Design review of the part built by this model. Coordinates are the model's own, in mm. A direction names the side the tool comes from. Give positions to 0.01 mm unless a question says otherwise; leave off trailing zeros. Order: outer loops, then holes, each group sorted by start corner. A loop starts at its lowest first (then second) coordinate and runs counter-clockwise, first axis right, second up. Notation, with made-up numbers: (61.25, 74) -> (105.25, 74) arc R19 ccw to (105.25, 107) -> close; hole circle Ø9 at (24, -11.5). An arc over 180 degrees is marked (long way). Return JSON: item names as keys, results as strings.
```python
from build123d import *
from build123d.topology import SkipClean

# Parameters (mm, degrees)
SKETCH2_R           = 31.369
BOSS_EXTRUDE1_DEPTH = 25.4
BOSS_EXTRUDE2_START = 125.476
BOSS_EXTRUDE2_DEPTH = 125.476
BOSS_EXTRUDE3_DEPTH = 49.022
SKETCH8_W           = 125.476
SKETCH8_H           = 49.022
BOSS_EXTRUDE4_DEPTH = 35.052
SKETCH9_W           = 125.476
SKETCH9_H           = 49.022
BOSS_EXTRUDE5_DEPTH = 35.052
SKETCH10_W          = 125.476
SKETCH10_H          = 35.052
BOSS_EXTRUDE6_DEPTH = 38.1
SKETCH12_W          = 125.476
SKETCH12_H          = 60.452
BOSS_EXTRUDE7_DEPTH = 52.324


with BuildPart() as part:
    # Sketch2 → Boss-Extrude1 (new body)
    with BuildSketch(Plane.YZ):
        with Locations(Location((0, 0, 0), (0, 0, 270))):
            Circle(SKETCH2_R)
    extrude(amount=BOSS_EXTRUDE1_DEPTH)

    # Sketch4 → Boss-Extrude2 (add)
    with SkipClean():  # the faces are left unmerged after this step: merging them gives an invalid solid
        with BuildSketch(Plane(origin=(0, 0, 0), x_dir=(0, -1, 0), z_dir=(-1, 0, 0)).offset(BOSS_EXTRUDE2_START)):
            with BuildLine():
                Line((31.369, 0), (31.369, 76.2))
                Line((31.369, 76.2), (-31.369, 76.2))
                Line((-31.369, 76.2), (-31.369, 0))
                ThreePointArc((-31.369, 0), (0, -31.369), (31.369, 0))
            make_face()
        extrude(amount=-BOSS_EXTRUDE2_DEPTH)

    # Sketch5 → Boss-Extrude3 (add)
    with SkipClean():  # the faces are left unmerged after this step: merging them gives an invalid solid
        with BuildSketch(Plane.XY.offset(76.2)):
            Polygon((0, 0), (0, 62.747251031), (-125.476, 62.747251031), (-125.476, -62.747251031), (0, -62.747251031), align=None)
        extrude(amount=BOSS_EXTRUDE3_DEPTH)

    # Sketch8 → Boss-Extrude4 (add)
    with SkipClean():  # the faces are left unmerged after this step: merging them gives an invalid solid
        with BuildSketch(Plane(origin=(0, 62.747251031, 0), x_dir=(-1, 0, 0), z_dir=(0, 1, 0))):
            with Locations((62.738, 100.711)):
                Rectangle(SKETCH8_W, SKETCH8_H)
        extrude(amount=BOSS_EXTRUDE4_DEPTH)

    # Sketch9 → Boss-Extrude5 (add)
    with SkipClean():  # the faces are left unmerged after this step: merging them gives an invalid solid
        with BuildSketch(Plane.XZ.offset(62.747251031)):
            with Locations((-62.738, 100.711)):
                Rectangle(SKETCH9_W, SKETCH9_H)
        extrude(amount=BOSS_EXTRUDE5_DEPTH)

    # Sketch10 → Boss-Extrude6 (add)
    with SkipClean():  # the faces are left unmerged after this step: merging them gives an invalid solid
        with BuildSketch(Plane.XY.offset(125.222)):
            with Locations((-62.738, 80.273251031)):
                Rectangle(SKETCH10_W, SKETCH10_H)
            with Locations((-62.738, -80.273251031)):
                Rectangle(SKETCH10_W, SKETCH10_H)
        extrude(amount=BOSS_EXTRUDE6_DEPTH)

    # Sketch12 → Boss-Extrude7 (add)
    with SkipClean():  # the faces are left unmerged after this step: merging them gives an invalid solid
        with BuildSketch(Plane.XY.offset(163.322)):
            with Locations((-62.738, 67.573251031)):
                Rectangle(SKETCH12_W, SKETCH12_H)
            with Locations((-62.738, -67.573251031)):
                Rectangle(SKETCH12_W, SKETCH12_H)
        extrude(amount=BOSS_EXTRUDE7_DEPTH)


solid = part.part
```
Item 1: Wall thickness on L1, parallel to Y at x = -32.5, z = 131.5; L2, parallel to Z at x = -24.5, y = 48.5; L3, parallel to Z at x = -113.5, y = -68.5: over which ranges is each line inside the solid? List them lowest first. Write a range as [from, to].
Result set:
{"L1": "y = [-97.8, -62.75], [62.75, 97.8]", "L2": "z = [76.2, 125.22], [163.32, 215.65]", "L3": "z = [76.2, 215.65]"}
Item 2: Add section C-C (x = -92). Give the boundary of the cut face in (y, z), plus the area to 3 significant figures.
Result set:
{"outline": "(-97.8, 76.2) -> (-31.37, 76.2) -> (-31.37, 0) arc R31.37 ccw to (31.37, 0) -> (31.37, 76.2) -> (97.8, 76.2) -> (97.8, 215.65) -> (37.35, 215.65) -> (37.35, 163.32) -> (62.75, 163.32) -> (62.75, 125.22) -> (-62.75, 125.22) -> (-62.75, 163.32) -> (-37.35, 163.32) -> (-37.35, 215.65) -> (-97.8, 215.65) -> close", "area": "24,900 mm^2"}
Item 3: Machinability: for faces 1 (the face through (-64, 31.369, 39)), 2 (the face through (-64, -31.369, 38)), 3 (the face through (-64, 37.347, 189)), 4 (the face through (-64, 62.747, 144)), which of the approach directions +Z, -Z, +X, -X, +Y, -Y give a long, thin tool a straight path to every point of the face, cutting with its end or side? Answer none if there is none.
Result set:
{"face 1": "-Z, +X, -X, +Y", "face 2": "-Z, +X, -X, -Y", "face 3": "+Z, +X, -X", "face 4": "+X, -X"}
Item 4: Add section A-A (y = -54.5). Give the boundary of the cut face in (x, z), plus the area to 3 significant figures.
Result set:
{"outline": "(-125.48, 76.2) -> (0, 76.2) -> (0, 125.22) -> (-125.48, 125.22) -> close; (-125.48, 163.32) -> (0, 163.32) -> (0, 215.65) -> (-125.48, 215.65) -> close", "area": "12,700 mm^2"}
Item 5: Add section B-B (z = 146.5). Give the boundary of the cut face in (x, y).
Result set:
{"outline": "(-125.48, -97.8) -> (0, -97.8) -> (0, -62.75) -> (-125.48, -62.75) -> close; (-125.48, 62.75) -> (0, 62.75) -> (0, 97.8) -> (-125.48, 97.8) -> close"}
Item 6: For pin 1 (7.5 mm diameter, centred on x = -57, y = -49, fed in from -Z); pin 2 (23 mm diameter, centred on x = -41, z = 49, fed in from -Y); pin 3 (3 mm diameter, centred on x = -83, z = 40, fed in from +Y), all flat-tipped, find the tip position at first contact; note any pin that passes through.
Result set:
{"pin 1": "stops at z = 76.2", "pin 2": "stops at y = -31.37", "pin 3": "stops at y = 31.37"}
Item 7: Add section D-D (y = 77). Give the boundary of the cut face in (x, z).
Result set:
{"outline": "(-125.48, 76.2) -> (0, 76.2) -> (0, 215.65) -> (-125.48, 215.65) -> close"}
Item 8: Mouldability with a two-part tool opening along Z and no side actions: class faces 5 (the face through (-64, -64, 76.2)), 6 (the face through (-64, -97.799, 147)), 7 (the face through (-64, 50, 163.322)) as released by +Z, released by -Z, zero draft, split by the parting line, or undercut.
Result set:
{"face 5": "released by -Z", "face 6": "zero draft", "face 7": "undercut"}
